The listing builds one solid part. Answer for the finished solid, in the listing's coordinates (mm). A direction names the side the tool comes from. Coordinates: 2 decimals unless noted, no trailing zeros. Order: outer loops, then holes, each group sorted by start corner. A loop starts at its lowest first (then second) coordinate and runs counter-clockwise, first axis right, second up. Notation, with made-up numbers: (27, 41) - (50, 41) arc R17 ccw to (50, 50) - close; hole circle Ø3 at (-2.5, -10). An arc over 180 degrees is marked (long way). One line per item, written item: value. Start each with the question number.
```python
from build123d import *

# Parameters (mm, degrees)
F2_T = -2
F3_R = 20


with BuildPart() as f1:
    # F0 (on Front) → F1 (revolve)
    with BuildSketch(Plane.XZ):
        Polygon((-32, -36.9929058894), (0, -36.9929058894), (0, 74.4539797306), (0, 82.0070941106), (-15.4507753317, 82.0070941106), (-32, 82.0070941106), align=None)
        with BuildLine():
            Line((-15.4507753317, 82.0070941106), (0, 82.0070941106))
            Line((0, 82.0070941106), (0, 132.6008036984))
            ThreePointArc((0, 132.6008036984), (-26.4501886014, 113.0223019318), (-15.4507753317, 82.0070941106))
        make_face()
    revolve(axis=Axis((0, 0, 47.8039489045), (0, 0, 1)))

    # F2
    f2_openings = [f1.faces().sort_by_distance(p)[0] for p in [
        (0, 0, -36.992906),
    ]]
    offset(amount=F2_T, openings=f2_openings, kind=Kind.INTERSECTION)

    # F3
    f3_edges = [f1.edges().sort_by_distance(p)[0] for p in [
        (30, 0, 80.007094),
    ]]
    fillet(f3_edges, radius=F3_R)


solid = f1.part
```
(1) The part is cut by section A-A on y = -23. Count the separate pieces of the cut face and the enclosed holes in it, plus the area to 3 significant figures.
(2) The part is cut by section C-C on z = -16.5. Determine the outline of the cut face in (x, y).
(3) Consider probe 1 along Y at (x, z) = (0, 27); probe 2 along Z at (x, y) = (9.5, -15); probe 3 along Z at (x, y) = (5.5, 17). Determine where each line is inside the solid, lowest interval first.
(4) For a pull along X with two mould halves and no side action, classify faces 3 (the face through (6.94, 31.24, 21.67)), 4 (the face through (29.97, -1.32, 10.83)), 5 (the face through (-9, -29, -36.993)) as pulls with the +X half, pulls with the -X half, needs draft (parallel to the pull), parting line crosses it, or undercut.
(5) The part is cut by section D-D on z = 108. Determine the outline of the cut face in (x, y).
(6) Flat-ended cylindrical pins translate along their axes: pin 1 Ø2 at (y, z) = (25.5, 0) entering from -X; pin 2 Ø12 at (x, z) = (-19, 109.5) entering from +Y; pin 3 Ø3 at (x, y) = (-25.5, -4.5) entering from -Z. Find the tip coordinate at first contact, or state that the pin passes through.
(7) For faces 1 (the face through (14, -8, 82.007)), 2 (the face through (7, 0, 80.007)), determine the directions among +Z, -Z, +X, -X, +Y, -Y from which every point of the face is accessible in a straight line to the end or side of a thin tool.
Completed:
1. separate pieces: 2
1. enclosed holes: 1
1. area: 1,430 mm2
2. outline: circle Ø64 at (0, 0); hole circle Ø60 at (0, 0)
3. probe 1: y = -32 to -30, 30 to 32
3. probe 2: z = 78.44 to 82.01, 83.74 to 86.42, 123.46 to 126.15
3. probe 3: z = 78.39 to 82.01, 83.84 to 86.53, 123.36 to 126.05
4. face 3: parting line crosses it
4. face 4: undercut
4. face 5: needs draft
5. outline: circle Ø54.97 at (0, 0); hole circle Ø50.95 at (0, 0)
6. pin 1: stops at x = -20.59
6. pin 2: stops at y = 24.12
6. pin 3: stops at z = 69.88
7. face 1: none
7. face 2: -Z
